The model under review builds one solid part; all positions refer to its coordinate system, in mm. A direction names the side the tool comes from. Give positions to 0.01 mm unless a question says otherwise; leave off trailing zeros. Order: outer loops, then holes, each group sorted by start corner. A loop starts at its lowest first (then second) coordinate and runs counter-clockwise, first axis right, second up. Notation, with made-up numbers: (28, 53.25) - (58, 53.25) arc R16 cw to (58, 61.25) - close; hole circle Ø3 at (38, 70). An arc over 180 degrees is marked (long way). Use a Markdown table: item, result. Add a question column.
```python
from build123d import *

# Parameters (mm, degrees)
BOSS_EXTRUDE1_DEPTH = 0.35
BOSS_EXTRUDE2_DEPTH = 0.7


with BuildPart() as part:
    # Sketch1 → Boss-Extrude1 (new, symmetric)
    with BuildSketch(Plane(origin=(0, 0, 0), x_dir=(1, 0, 0), z_dir=(0, 1, 0))):
        with BuildLine():
            Line((70.992084628, 5.693181902), (83.950482552, 6.732375453))
            ThreePointArc((83.950482552, 6.732375453), (0, -84.22), (-83.950482552, 6.732375453))
            Line((-83.950482552, 6.732375453), (-70.992084628, 5.693181902))
            ThreePointArc((-70.992084628, 5.693181902), (0, -71.22), (70.992084628, 5.693181902))
        make_face()
    extrude(amount=BOSS_EXTRUDE1_DEPTH, both=True)

    # Sketch2 → Boss-Extrude2 (add)
    with BuildSketch(Plane(origin=(0, 0.35, 0), x_dir=(1, 0, 0), z_dir=(0, 1, 0))):
        with BuildLine():
            Line((71.979704881, 5.772383714), (82.964261813, 6.653285874))
            Line((82.964261813, 6.653285874), (82.836871628, 7.976283525))
            Line((82.836871628, 7.976283525), (83.832267826, 8.072129277))
            ThreePointArc((83.832267826, 8.072129277), (82.940508959, 14.624649523), (81.537394273, 21.087003941))
            Line((81.537394273, 21.087003941), (68.951474948, 17.832063889))
            ThreePointArc((68.951474948, 17.832063889), (70.13800817, 12.367223213), (70.892117248, 6.826134494))
            Line((70.892117248, 6.826134494), (71.887513446, 6.921980247))
            Line((71.887513446, 6.921980247), (71.979704881, 5.772383714))
        make_face()
        with BuildLine():
            Line((-82.964261813, 6.653285874), (-71.979704881, 5.772383714))
            Line((-71.979704881, 5.772383714), (-71.887513446, 6.921980247))
            Line((-71.887513446, 6.921980247), (-70.892117248, 6.826134494))
            ThreePointArc((-70.892117248, 6.826134494), (-70.13800817, 12.367223213), (-68.951474948, 17.832063889))
            Line((-68.951474948, 17.832063889), (-81.537394273, 21.087003941))
            ThreePointArc((-81.537394273, 21.087003941), (-82.940508959, 14.624649523), (-83.832267826, 8.072129277))
            Line((-83.832267826, 8.072129277), (-82.836871628, 7.976283525))
            Line((-82.836871628, 7.976283525), (-82.964261813, 6.653285874))
        make_face()
    extrude(amount=-BOSS_EXTRUDE2_DEPTH)


solid = part.part
```
Q1. We need section A-A (z = 0). Write out the cut boundary in (x, y).
Q2. We need section C-C (x = 0). Write out the cut boundary in (y, z), plus the area to 3 significant figures.
Q3. We need section D-D (z = 37). Write out the cut boundary in (x, y).
Q4. Machinability: for faces 4 (the flat face through (12.9, -0.35, 70.3)), 5 (the flat face through (75.33, 0, -19.48)), which of the approach directions +Z, -Z, +X, -X, +Y, -Y give a long, thin tool a straight path to every point of the face, cutting with its end or side? Answer none if there is none.
Q5. Wall thickness on probe 1 along X at (y, z) = (-0.1, 0); probe 2 along X at (y, z) = (0.2, 24.5); probe 3 along Z at (x, y) = (0, -0.1): over which ranges is each line inside the solid? List them lowest first.
Q6. We need section B-B (y = 0.2). Write out the cut boundary in (x, z), plus the area to 3 significant figures.
Q7. Draft analysis for pull direction X (two halves, no side actions). For faces 1 (the cylindrical face through (1.9, 0, 84.2)), 2 (the cylindrical face through (-1.65, 0, 71.2)), 3 (the flat face through (12.9, 0.35, 70.3)), state which applies: pulls with the +X half, pulls with the -X half, needs draft (parallel to the pull), parting line crosses it, or undercut.
Here are the results:
| question | item | result |
|---|---|---|
| 1 | outline | (-84.22, -0.35) - (-71.22, -0.35) - (-71.22, 0.35) - (-84.22, 0.35) - close; (71.22, -0.35) - (84.22, -0.35) - (84.22, 0.35) - (71.22, 0.35) - close |
| 2 | outline | (-0.35, 71.22) - (0.35, 71.22) - (0.35, 84.22) - (-0.35, 84.22) - close |
| 2 | area | 9.10 mm2 |
| 3 | outline | (-75.66, -0.35) - (-60.85, -0.35) - (-60.85, 0.35) - (-75.66, 0.35) - close; (60.85, -0.35) - (75.66, -0.35) - (75.66, 0.35) - (60.85, 0.35) - close |
| 4 | face 4 | +Z, -Z, +X, -X, -Y |
| 4 | face 5 | -Z, +Y, -Y |
| 5 | probe 1 | -84.22 to -71.22, 71.22 to 84.22 |
| 5 | probe 2 | -80.58 to -66.87, 66.87 to 80.58 |
| 5 | probe 3 | 71.22 to 84.22 |
| 6 | outline | (-83.95, -6.73) - (-82.96, -6.65) - (-82.84, -7.98) - (-83.83, -8.07) arc R84.22 ccw to (-81.54, -21.09) - (-68.95, -17.83) arc R71.22 cw to (-70.89, -6.83) - (-71.89, -6.92) - (-71.98, -5.77) - (-70.99, -5.69) arc R71.22 cw (long way) to (70.99, -5.69) - (71.98, -5.77) - (71.89, -6.92) - (70.89, -6.83) arc R71.22 cw to (68.95, -17.83) - (81.54, -21.09) arc R84.22 ccw to (83.83, -8.07) - (82.84, -7.98) - (82.96, -6.65) - (83.95, -6.73) arc R84.22 ccw (long way) to start |
| 6 | area | 3,680 mm2 |
| 7 | face 1 | parting line crosses it |
| 7 | face 2 | undercut |
| 7 | face 3 | needs draft |
